Verification items for the finished model (mm, model axes). Round coordinates to 2 decimals unless told otherwise and drop trailing zeros. Loops run counter-clockwise (first coordinate to the right, second up) from the corner with the lowest first, then second, coordinate; pieces in that order, holes last. Notation, with made-up numbers: M -5.5,61.5 L 47.5,61.5 A15 ccw 47.5,88.5 Z; hole C 57.5,49 d2. An arc over 180 degrees is marked long. One line per item, written item: value.
from build123d import *

# Parameters (mm, degrees)
SKETCH1_W                                    = 20
SKETCH1_H                                    = 11
BOSS_EXTRUDE1_DEPTH                          = 520
CUT_EXTRUDE1_DEPTH                           = 521
CBORE_FOR_SOCKET_HEAD_CAP_SCREW1_D           = 6
CBORE_FOR_SOCKET_HEAD_CAP_SCREW1_CBORE_D     = 9.5
CBORE_FOR_SOCKET_HEAD_CAP_SCREW1_CBORE_DEPTH = 5.5
LPATTERN1_COUNT                              = 9
LPATTERN1_PITCH                              = 60
CHAMFER1_SIZE                                = 0.3
CHAMFER2_SIZE                                = 0.5


with BuildPart() as part:
    # Sketch1 → Boss-Extrude1 (new body)
    with BuildSketch(Plane(origin=(-20, 0, 0), x_dir=(0, 0, -1), z_dir=(1, 0, 0))):
        with Locations((0, 5.5)):
            Rectangle(SKETCH1_W, SKETCH1_H)
    extrude(amount=BOSS_EXTRUDE1_DEPTH)

    # Sketch2 → Cut-Extrude1 (cut, through all)
    with BuildSketch(Plane(origin=(-20, 0, 0), x_dir=(0, 0, -1), z_dir=(1, 0, 0))):
        with BuildLine():
            Line((10, 10.221039482), (9.455259378, 9.911421591))
            ThreePointArc((9.455259378, 9.911421591), (9.0228024, 9.564639684), (8.720500078, 9.1))
            Line((8.720500078, 9.1), (7.5, 9.1))
            Line((7.5, 9.1), (7.5, 7.9))
            Line((7.5, 7.9), (8.724976489, 7.9))
            ThreePointArc((8.724976489, 7.9), (9.018551739, 7.450071616), (9.434780564, 7.110401858))
            Line((9.434780564, 7.110401858), (10, 6.778960518))
            Line((10, 6.778960518), (10, 10.221039482))
        make_face()
        with BuildLine():
            Line((-10, 10.221039482), (-10, 6.778960518))
            Line((-10, 6.778960518), (-9.434780564, 7.110401858))
            ThreePointArc((-9.434780564, 7.110401858), (-9.018551739, 7.450071616), (-8.724976489, 7.9))
            Line((-8.724976489, 7.9), (-7.5, 7.9))
            Line((-7.5, 7.9), (-7.5, 9.1))
            Line((-7.5, 9.1), (-8.720500078, 9.1))
            ThreePointArc((-8.720500078, 9.1), (-9.0228024, 9.564639684), (-9.455259378, 9.911421591))
            Line((-9.455259378, 9.911421591), (-10, 10.221039482))
        make_face()
    extrude(amount=CUT_EXTRUDE1_DEPTH, mode=Mode.SUBTRACT)

    # CBORE for Socket Head Cap Screw1 (through all)
    with Locations(Plane(origin=(0, 11, 0), x_dir=(1, 0, 0), z_dir=(0, 1, 0))):
        with Locations((0, 0)):
            cbore_for_socket_head_cap_screw1 = CounterBoreHole(CBORE_FOR_SOCKET_HEAD_CAP_SCREW1_D / 2, CBORE_FOR_SOCKET_HEAD_CAP_SCREW1_CBORE_D / 2, CBORE_FOR_SOCKET_HEAD_CAP_SCREW1_CBORE_DEPTH)

    # LPattern1: CBORE for Socket Head Cap Screw1 ×9
    with Locations(*[(i * LPATTERN1_PITCH, 0, 0) for i in range(1, LPATTERN1_COUNT)]):
        add(cbore_for_socket_head_cap_screw1, mode=Mode.SUBTRACT)

    # Chamfer1
    chamfer1_edges = [part.edges().sort_by_distance(p)[0] for p in [
        (240, 11, 10),
        (240, 11, -10),
    ]]
    chamfer(chamfer1_edges, length=CHAMFER1_SIZE)

    # Chamfer2
    chamfer2_edges = [part.edges().sort_by_distance(p)[0] for p in [
        (240, 0, -10),
        (240, 0, 10),
    ]]
    chamfer(chamfer2_edges, length=CHAMFER2_SIZE)


solid = part.part
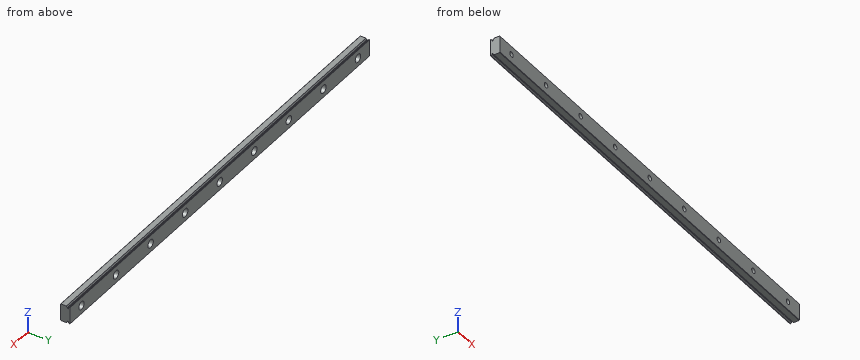
(1) Sectioned sample at B-B on y = 3. Count the separate pieces of the cut face and the enclosed holes in it, and give its area (3 significant figures).
Completed:
separate pieces: 1
enclosed holes: 9
area: 10,100 mm^2
(2) Thickness scan on L1, parallel to Z at x = 0, y = 2.5; L2, parallel to Y at x = 93.5, z = -8; L3, parallel to Z at x = 240, y = 8.1. Record the ranges inside material, lowest first. Write a range as from..to.
Completed:
L1: z = -10..-3, 3..10
L2: y = 0..7.9, 9.1..11
L3: z = -7.5..-4.75, 4.75..7.5
(3) Sectioned sample at A-A on x = 20.5. Enter the section's corners in (y, z), and give its area (3 significant figures).
Completed:
outline: M 0,-9.5 L 0.5,-10 L 6.78,-10 L 7.11,-9.43 A1.75 cw 7.9,-8.72 L 7.9,-7.5 L 9.1,-7.5 L 9.1,-8.72 A1.75 cw 9.91,-9.46 L 10.22,-10 L 10.7,-10 L 11,-9.7 L 11,9.7 L 10.7,10 L 10.22,10 L 9.91,9.46 A1.75 cw 9.1,8.72 L 9.1,7.5 L 7.9,7.5 L 7.9,8.72 A1.75 cw 7.11,9.43 L 6.78,10 L 0.5,10 L 0,9.5 Z
area: 210 mm^2
(4) Depth check by flat-ended pin: pin 1 Ø8.5 at (x, z) = (0, 0) entering from +Y; pin 2 Ø1 at (x, y) = (362.5, 8.5) entering from -Z. Enter the tip coordinate at first touch or a pass-through.
Completed:
pin 1: stops at y = 5.5
pin 2: stops at z = -7.5
